Model file for the job. Use its own axes, mm. Face numbers are marked on the shaded views. A direction names the side the tool comes from. Coordinates: 2 decimals unless noted, no trailing zeros. Write each loop counter-clockwise with the first axis right and the second up, starting at its lowest first coordinate (ties: lowest second). Pieces come first, ordered by that corner, then holes. Notation, with made-up numbers: M -37,87.5 L -18,87.5 A7 ccw -18,100.5 Z; hole C -23.5,89.25 d3. An arc over 180 degrees is marked long. One line per question, with ' | ' between items. Start each with the question number.
(1) Flat gauge pins, fed straight in: pin 1 Ø6 at (x, z) = (-14, -5.5) entering from +Y; pin 2 Ø1.5 at (x, y) = (2, 106.5) entering from +Z; pin 3 Ø3 at (x, z) = (6.5, -3) entering from +Y. Where does each tip first touch, or does it go through?
(2) Cut at C-C (y = 33). Write the cut outline in (x, z), plus the area to 3 significant figures.
(3) Cut at A-A (x = 10). Write the cut outline in (y, z), plus the area to 3 significant figures.
(4) Tool access for the marked faces 1 and 2: list every direction of +Z, -Z, +X, -X, +Y, -Y with a clear straight run to the whole face (end or side of a thin tool).
(5) Wall check: probe 1 along Z at (x, y) = (-14, 4); probe 2 along Z at (x, y) = (4.25, 102.5); probe 3 along Y at (x, z) = (-11.75, -8). Give the ranges that are in metal, low to high.
(6) Cut at B-B (x = -14). Write the cut outline in (y, z), plus the area to 3 significant figures.
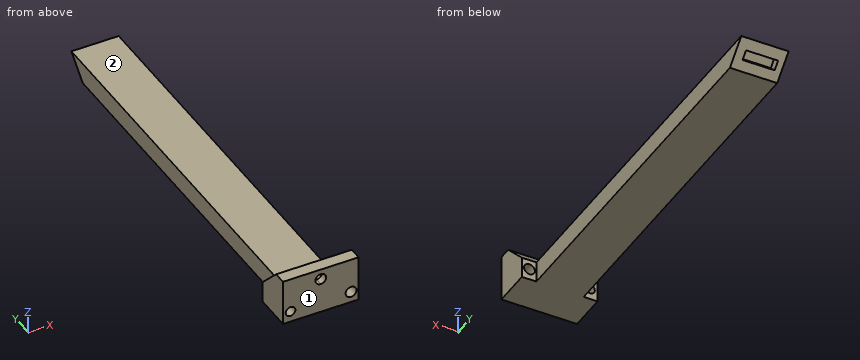
from build123d import *

# Parameters (mm, degrees)
BOSS_EXTRUDE1_DEPTH = 15
CHAMFER1_SIZE       = 10
SKETCH2_R           = 3.544680495
CUT_EXTRUDE1_DEPTH  = 12
SKETCH3_W           = 18.759195859
SKETCH3_H           = 8.35
BOSS_EXTRUDE2_DEPTH = 150
CUT_EXTRUDE2_DEPTH  = 150
SKETCH5_W           = 12.715839202
SKETCH5_H           = 3.591790086
CUT_EXTRUDE3_DEPTH  = 4


with BuildPart() as part:
    # Sketch1 → Boss-Extrude1 (new body)
    with BuildSketch(Plane(origin=(0, 0, 0), x_dir=(1, 0, 0), z_dir=(0, 1, 0))):
        with BuildLine():
            Line((13, 8.926911476), (-2, 8.926911476))
            Line((-2, 8.926911476), (-2, 4.542283032))
            Line((-2, 4.542283032), (7.841609066, 4.542283032))
            ThreePointArc((7.841609066, 4.542283032), (10, 6.700673966), (12.158390934, 4.542283032))
            Line((12.158390934, 4.542283032), (13, 4.542283032))
            Line((13, 4.542283032), (13, 8.926911476))
        make_face()
        with BuildLine():
            Line((-2, 4.542283032), (-2, 8.926911476))
            Line((-2, 8.926911476), (-17, 8.926911476))
            Line((-17, 8.926911476), (-17, 4.542283032))
            Line((-17, 4.542283032), (-15.919451213, 4.542283032))
            ThreePointArc((-15.919451213, 4.542283032), (-14, 6.461734245), (-12.080548787, 4.542283032))
            Line((-12.080548787, 4.542283032), (-2, 4.542283032))
        make_face()
        with BuildLine():
            Line((-2, -3.130873366), (-2, 4.542283032))
            Line((-2, 4.542283032), (-12.080548787, 4.542283032))
            ThreePointArc((-12.080548787, 4.542283032), (-14, 2.622831819), (-15.919451213, 4.542283032))
            Line((-15.919451213, 4.542283032), (-17, 4.542283032))
            Line((-17, 4.542283032), (-17, -9.423088524))
            Line((-17, -9.423088524), (-2, -9.423088524))
            Line((-2, -9.423088524), (-2, -7.40597744))
            ThreePointArc((-2, -7.40597744), (-4.137552037, -5.268425403), (-2, -3.130873366))
        make_face()
        with BuildLine():
            Line((7.841609066, 4.542283032), (-2, 4.542283032))
            Line((-2, 4.542283032), (-2, -3.130873366))
            ThreePointArc((-2, -3.130873366), (-0.488522459, -3.756947863), (0.137552037, -5.268425403))
            ThreePointArc((0.137552037, -5.268425403), (-0.488522459, -6.779902944), (-2, -7.40597744))
            Line((-2, -7.40597744), (-2, -9.423088524))
            Line((-2, -9.423088524), (13, -9.423088524))
            Line((13, -9.423088524), (13, 4.542283032))
            Line((13, 4.542283032), (12.158390934, 4.542283032))
            ThreePointArc((12.158390934, 4.542283032), (10, 2.383892098), (7.841609066, 4.542283032))
        make_face()
    extrude(amount=BOSS_EXTRUDE1_DEPTH)

    # Chamfer1
    # the kernel refuses this chamfer: 10 mm, written as the material it takes off along each edge
    with BuildSketch(Plane(origin=(-42.71682988, 15, 9.423088524), x_dir=(0, -0.9996219169112968, 0.027495876610586317), z_dir=(1, 0, 0))) as chamfer1_piece_1:
        Polygon((CHAMFER1_SIZE * 0.999621916911, CHAMFER1_SIZE * 0.0274958766106), (-CHAMFER1_SIZE * 0.0274958766106, CHAMFER1_SIZE * 0.999621916911), (0, 0), align=None)
    extrude(amount=81.433659759, mode=Mode.SUBTRACT)

    # Sketch2 → Cut-Extrude1 (cut)
    with BuildSketch(Plane(origin=(0, 15, 0), x_dir=(1, 0, 0), z_dir=(0, 1, 0))):
        with Locations(Location((-2, -5.268425403, 0), (0, 0, 270))):
            Circle(SKETCH2_R)
    extrude(amount=-CUT_EXTRUDE1_DEPTH, mode=Mode.SUBTRACT)

    # Sketch3 → Boss-Extrude2 (add)
    with BuildSketch(Plane(origin=(0, 15, 0), x_dir=(1, 0, 0), z_dir=(0, 1, 0))):
        with Locations((-2.146940407, 4.751911476)):
            Rectangle(SKETCH3_W, SKETCH3_H)
    extrude(amount=BOSS_EXTRUDE2_DEPTH)

    # Sketch4 → Cut-Extrude2 (cut)
    with BuildSketch(Plane(origin=(7.232657523, 0, 0), x_dir=(0, 0, -1), z_dir=(1, 0, 0))):
        Polygon((0.576911476, 165), (8.926911476, 156.65), (8.926911476, 165), align=None)
    extrude(amount=-CUT_EXTRUDE2_DEPTH, mode=Mode.SUBTRACT)

    # Sketch5 → Cut-Extrude3 (cut)
    with BuildSketch(Plane(origin=(0, 82.788455738, -82.788455738), x_dir=(1, 0, 0), z_dir=(0, 0.707106781186556, -0.707106781186539))):
        with Locations((-2.621419411, -110.225300743)):
            Rectangle(SKETCH5_W, SKETCH5_H)
    extrude(amount=-CUT_EXTRUDE3_DEPTH, mode=Mode.SUBTRACT)


solid = part.part
Filled in:
1) pin 1: y = 161.77 | pin 2: z = -0.58 | pin 3: y = 164.08
2) outline: M -11.53,-8.93 L 7.23,-8.93 L 7.23,-0.58 L -11.53,-0.58 Z | area: 157 mm²
3) outline: M 0,-8.93 L 15,-8.93 L 15,-6.7 L 0,-6.7 Z; M 0,-2.38 L 15,-2.38 L 15,-0.58 L 5,9.42 L 0,9.42 Z | area: 160 mm²
4) face 1: +Z, -Z, +X, -X, -Y | face 2: +Z, +X, -X, +Y
5) probe 1: -8.93 to -6.46, -2.62 to 9.42 | probe 2: -8.93 to -0.58 | probe 3: 0 to 15
6) outline: M 0,-8.93 L 15,-8.93 L 15,-6.46 L 0,-6.46 Z; M 0,-2.62 L 15,-2.62 L 15,-0.58 L 5,9.42 L 0,9.42 Z | area: 168 mm²
